from build123d import *

# Parameters (mm, degrees)
WIRING_SLOTS_AND_DECK_MOUNTS_PROFILE_W   = 109
WIRING_SLOTS_AND_DECK_MOUNTS_PROFILE_H   = 192
WIRING_SLOTS_AND_DECK_MOUNTS_PROFILE_R   = 2.2
WIRING_SLOTS_AND_DECK_MOUNTS_PROFILE_R_2 = 1.75
WIRING_SLOTS_AND_DECK_MOUNTS_DEPTH       = 3


with BuildPart() as part:
    # Wiring slots and deck mounts profile → Wiring slots and deck mounts (new body)
    with BuildSketch(Plane.XY):
        with Locations((-0.5, 0)):
            Rectangle(WIRING_SLOTS_AND_DECK_MOUNTS_PROFILE_W, WIRING_SLOTS_AND_DECK_MOUNTS_PROFILE_H)
        with Locations((-37, -81)):
            Circle(WIRING_SLOTS_AND_DECK_MOUNTS_PROFILE_R, mode=Mode.SUBTRACT)
        with Locations((-37, 81)):
            Circle(WIRING_SLOTS_AND_DECK_MOUNTS_PROFILE_R, mode=Mode.SUBTRACT)
        with Locations((30, -81)):
            Circle(WIRING_SLOTS_AND_DECK_MOUNTS_PROFILE_R, mode=Mode.SUBTRACT)
        with Locations((30, 81)):
            Circle(WIRING_SLOTS_AND_DECK_MOUNTS_PROFILE_R, mode=Mode.SUBTRACT)
        with Locations((-22, -83)):
            Circle(WIRING_SLOTS_AND_DECK_MOUNTS_PROFILE_R_2, mode=Mode.SUBTRACT)
        with Locations((-22, 39)):
            Circle(WIRING_SLOTS_AND_DECK_MOUNTS_PROFILE_R_2, mode=Mode.SUBTRACT)
        with Locations((-22, -39)):
            Circle(WIRING_SLOTS_AND_DECK_MOUNTS_PROFILE_R_2, mode=Mode.SUBTRACT)
        with Locations((-22, 83)):
            Circle(WIRING_SLOTS_AND_DECK_MOUNTS_PROFILE_R_2, mode=Mode.SUBTRACT)
        with Locations((22, -83)):
            Circle(WIRING_SLOTS_AND_DECK_MOUNTS_PROFILE_R_2, mode=Mode.SUBTRACT)
        with Locations((22, 39)):
            Circle(WIRING_SLOTS_AND_DECK_MOUNTS_PROFILE_R_2, mode=Mode.SUBTRACT)
        with Locations((22, -39)):
            Circle(WIRING_SLOTS_AND_DECK_MOUNTS_PROFILE_R_2, mode=Mode.SUBTRACT)
        with Locations((22, 83)):
            Circle(WIRING_SLOTS_AND_DECK_MOUNTS_PROFILE_R_2, mode=Mode.SUBTRACT)
        with BuildLine():
            Line((-41, -4), (-17, -4))
            ThreePointArc((-17, -4), (-13, 0), (-17, 4))
            Line((-17, 4), (-41, 4))
            ThreePointArc((-41, 4), (-45, 0), (-41, -4))
        make_face(mode=Mode.SUBTRACT)
        with BuildLine():
            Line((13, -4), (37, -4))
            ThreePointArc((37, -4), (41, 0), (37, 4))
            Line((37, 4), (13, 4))
            ThreePointArc((13, 4), (9, 0), (13, -4))
        make_face(mode=Mode.SUBTRACT)
    extrude(amount=WIRING_SLOTS_AND_DECK_MOUNTS_DEPTH)


solid = part.part
Build history of the part. All positions in model axes, mm. A direction names the side the tool comes from. Give positions to 0.01 mm unless a question says otherwise; leave off trailing zeros. Answer in a Markdown table with one row per item.
Item 1: Tool access for faces 3 (the cylindrical face through (9, 0, 1)), 4 (the flat face through (-1, 1, 0)): list every direction of +Z, -Z, +X, -X, +Y, -Y with a clear straight run to the whole face (end or side of a thin tool).
Findings below:
| item | result |
|---|---|
| face 3 | +Z, -Z |
| face 4 | -Z, +X, -X, +Y, -Y |
Item 2: Slice it at A-A on z = 1.6. Give the number of separate pieces and of enclosed holes in the cut face, plus the area to 3 significant figures.
Findings below:
| item | result |
|---|---|
| separate pieces | 1 |
| enclosed holes | 14 |
| area | 20,300 mm² |
Item 3: Mould opens along X. For faces 1 (the cylindrical face through (28.38, 82.49, 1.48)), 2 (the flat face through (-1, 1, 3)) say: pulls with the +X half, pulls with the -X half, needs draft (parallel to the pull), parting line crosses it, or undercut.
Findings below:
| item | result |
|---|---|
| face 1 | undercut |
| face 2 | needs draft |
Item 4: Probe line 1 along Y through (x, z) = (-22, 2.1); line 2 along X through (y, z) = (-83, 1.35); line 3 along Y through (x, z) = (29, 0.3). List the from-to ranges inside material, lowest first. Write a range as [from, to].
Findings below:
| item | result |
|---|---|
| line 1 | y = [-96, -84.75], [-81.25, -40.75], [-37.25, -4], [4, 37.25], [40.75, 81.25], [84.75, 96] |
| line 2 | x = [-55, -37.92], [-36.08, -23.75], [-20.25, 20.25], [23.75, 29.08], [30.92, 54] |
| line 3 | y = [-96, -82.96], [-79.04, -4], [4, 79.04], [82.96, 96] |
